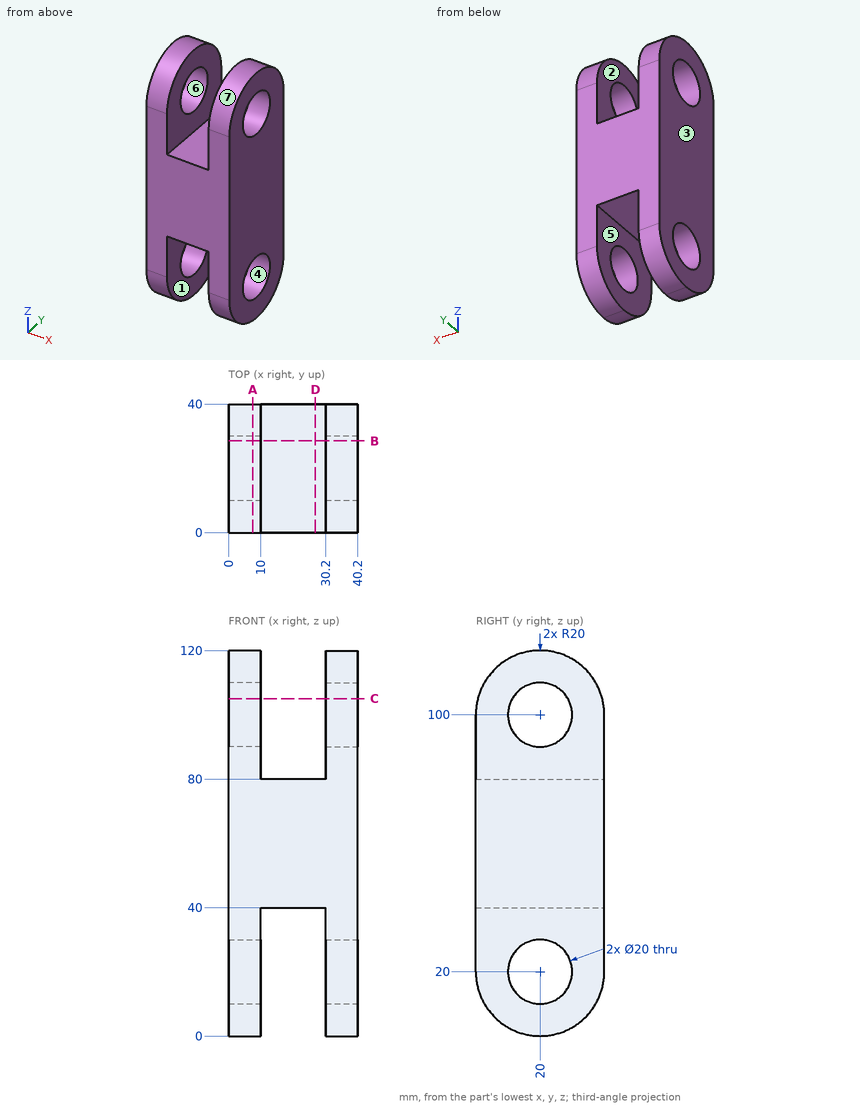
Study the drawing (mm; zero at the part's minimum x, y, z) and answer. A direction names the side the tool comes from. Coordinates: 2 decimals unless noted, no trailing zeros. Write each loop counter-clockwise with the first axis right and the second up, starting at its lowest first coordinate (ties: lowest second). Pieces come first, ordered by that corner, then holes. Notation, with made-up numbers: (39, 62.25) - (97, 62.25) arc R18 ccw to (97, 91.25) - close; hole circle Ø5 at (-9.5, -6). An arc over 180 degrees is marked (long way). Return JSON: item names as keys, results as strings. Group by question number.
1. A cutting plane is placed at D-D, the plane x = 27. Determine the outline of the cut face in (y, z).
2. Which of the six approach directions +Z, -Z, +X, -X, +Y, -Y give full straight-line access (tool end or side, diameter ignored) to the marked faces 1, 2 and 3?
3. Determine the mould class of the marked faces 4, 5, 6 and 7 for opening direction Z: released by +Z, released by -Z, zero draft, split by the parting line, or undercut.
4. Straight lines are drawn through the part: L1, parallel to Z at x = 33.75, y = 20; L2, parallel to X at y = 5.5, z = 39.5; L3, parallel to Z at x = 2.5, y = 12. For each, find the intervals that lie inside material, in ascending order.
5. A cutting plane is placed at A-A, the plane x = 7.5. Give the number of separate pieces and of enclosed holes in the cut face, plus the area to 3 significant figures.
6. A cutting plane is placed at B-B, the plane y = 28.5. Determine the outline of the cut face in (x, z).
7. A cutting plane is placed at C-C, the plane z = 105. Determine the outline of the cut face in (x, y).
8. Given pin 1 (5 mm diameter, centred on x = 32.5, y = 23, fed in from -Z); pin 2 (3 mm diameter, centred on x = 33, y = 8, fed in from -Z); pin 3 (22 mm diameter, centred on x = 18.5, y = 21, fed in from +Z), each flat-ended and moving along its own axis, determine where each tip first touches the part or whether it passes through.
Ans:
{
 "1": {"outline": "(0, 40) - (40, 40) - (40, 80) - (0, 80) - close"},
 "2": {"face 1": "-Z, +Y, -Y", "face 2": "+Z, +Y, -Y", "face 3": "+Z, -Z, -X, +Y, -Y"},
 "3": {"face 4": "undercut", "face 5": "zero draft", "face 6": "undercut", "face 7": "released by +Z"},
 "4": {"L1": "0 to 10, 30 to 90, 110 to 120", "L2": "0 to 10, 30.2 to 40.2", "L3": "1.67 to 14, 26 to 94, 106 to 118.33"},
 "5": {"separate pieces": "1", "enclosed holes": "2", "area": "3,830 mm²"},
 "6": {"outline": "(0, 1.9) - (10, 1.9) - (10, 14.73) - (0, 14.73) - close; (0, 25.27) - (10, 25.27) - (10, 40) - (30.2, 40) - (30.2, 25.27) - (40.2, 25.27) - (40.2, 94.73) - (30.2, 94.73) - (30.2, 80) - (10, 80) - (10, 94.73) - (0, 94.73) - close; (0, 105.27) - (10, 105.27) - (10, 118.1) - (0, 118.1) - close; (30.2, 1.9) - (40.2, 1.9) - (40.2, 14.73) - (30.2, 14.73) - close; (30.2, 105.27) - (40.2, 105.27) - (40.2, 118.1) - (30.2, 118.1) - close"},
 "7": {"outline": "(0, 0.64) - (10, 0.64) - (10, 11.34) - (0, 11.34) - close; (0, 28.66) - (10, 28.66) - (10, 39.36) - (0, 39.36) - close; (30.2, 0.64) - (40.2, 0.64) - (40.2, 11.34) - (30.2, 11.34) - close; (30.2, 28.66) - (40.2, 28.66) - (40.2, 39.36) - (30.2, 39.36) - close"},
 "8": {"pin 1": "z = 0.01", "pin 2": "z = 2.98", "pin 3": "z = 120"}
}
